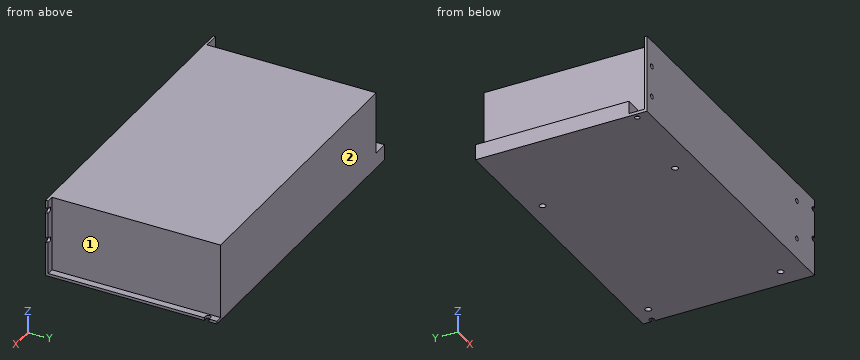
from build123d import *

# Parameters (mm, degrees)
SKETCH_1_W          = 200
SKETCH_1_H          = 110
EXTRUDE_1_DEPTH     = 50
SKETCH_2_R          = 2
CUT_EXTRUDE_1_DEPTH = 10
SKETCH_3_W          = 10
SKETCH_3_H          = 108.5
CUT_EXTRUDE_2_DEPTH = 40
SKETCH_6_W          = 4.5
SKETCH_6_H          = 48.2
CUT_EXTRUDE_5_DEPTH = 108.2
SKETCH_4_R          = 1.5
CUT_EXTRUDE_3_DEPTH = 10
SKETCH_5_R          = 1.6
CUT_EXTRUDE_4_DEPTH = 10
SKETCH_7_W          = 10
SKETCH_7_H          = 10
CUT_EXTRUDE_6_DEPTH = 8.2
SKETCH_8_R          = 1.6
CUT_EXTRUDE_7_DEPTH = 1.8


with BuildPart() as part:
    # 草图1 → 拉伸1 (new body)
    with BuildSketch(Plane.XY):
        with Locations((-22.033224223, 5.842062193)):
            Rectangle(SKETCH_1_W, SKETCH_1_H)
    extrude(amount=EXTRUDE_1_DEPTH)

    # 草图2 → 切除-拉伸1 (cut)
    with BuildSketch(Plane.XY):
        with Locations((-60.533224223, 50.842062193)):
            Circle(SKETCH_2_R)
        with Locations((65.466775777, 50.842062193)):
            Circle(SKETCH_2_R)
        with Locations((-60.533224223, -34.157937807)):
            Circle(SKETCH_2_R)
        with Locations((65.466775777, -34.157937807)):
            Circle(SKETCH_2_R)
    extrude(amount=CUT_EXTRUDE_1_DEPTH, mode=Mode.SUBTRACT)

    # 草图3 → 切除-拉伸2 (cut)
    with BuildSketch(Plane.XY.offset(50)):
        with Locations((-117.033224223, 6.592062193)):
            Rectangle(SKETCH_3_W, SKETCH_3_H)
    extrude(amount=-CUT_EXTRUDE_2_DEPTH, mode=Mode.SUBTRACT)

    # 草图6 → 切除-拉伸5 (cut)
    with BuildSketch(Plane(origin=(0, 60.842062193, 0), x_dir=(-1, 0, 0), z_dir=(0, 1, 0))):
        with Locations((-75.716775777, 25.9)):
            Rectangle(SKETCH_6_W, SKETCH_6_H)
    extrude(amount=-CUT_EXTRUDE_5_DEPTH, mode=Mode.SUBTRACT)

    # 草图4 → 切除-拉伸3 (cut)
    with BuildSketch(Plane.XZ.offset(49.157937807)):
        with Locations(Location((-116.033224223, 13, 0), (0, 0, 270))):
            Circle(SKETCH_4_R)
        with Locations(Location((56.966775777, 13, 0), (0, 0, 270))):
            Circle(SKETCH_4_R)
        with Locations(Location((56.966775777, 38, 0), (0, 0, 270))):
            Circle(SKETCH_4_R)
    extrude(amount=-CUT_EXTRUDE_3_DEPTH, mode=Mode.SUBTRACT)

    # 草图5 → 切除-拉伸4 (cut)
    with BuildSketch(Plane.XZ.offset(49.157937807)):
        with Locations(Location((-116.033224223, 33, 0), (0, 0, 270))):
            Circle(SKETCH_5_R)
        with BuildLine():
            Line((77.966775777, 45), (77.966775777, 41.8))
            Line((77.966775777, 41.8), (76.666775777, 41.8))
            ThreePointArc((76.666775777, 41.8), (75.066775777, 43.4), (76.666775777, 45))
            Line((76.666775777, 45), (77.966775777, 45))
        make_face()
        with BuildLine():
            Line((77.966775777, 22.1), (76.666775777, 22.1))
            ThreePointArc((76.666775777, 22.1), (75.066775777, 23.7), (76.666775777, 25.3))
            Line((76.666775777, 25.3), (77.966775777, 25.3))
            Line((77.966775777, 25.3), (77.966775777, 22.1))
        make_face()
    extrude(amount=-CUT_EXTRUDE_4_DEPTH, mode=Mode.SUBTRACT)

    # 草图7 → 切除-拉伸6 (cut)
    with BuildSketch(Plane.XY.offset(10)):
        with Locations((-117.033224223, -42.657937807)):
            Rectangle(SKETCH_7_W, SKETCH_7_H)
    extrude(amount=-CUT_EXTRUDE_6_DEPTH, mode=Mode.SUBTRACT)

    # 草图8 → 切除-拉伸7 (cut)
    with BuildSketch(Plane(origin=(0, 0, 0), x_dir=(-1, 0, 0), z_dir=(0, 0, -1))):
        with Locations((118.533224223, -41.157937807)):
            Circle(SKETCH_8_R)
        with BuildLine():
            Line((-77.966775777, 55.942062193), (-76.166775777, 55.942062193))
            ThreePointArc((-76.166775777, 55.942062193), (-74.566775777, 54.342062193), (-76.166775777, 52.742062193))
            Line((-76.166775777, 52.742062193), (-77.966775777, 52.742062193))
            Line((-77.966775777, 52.742062193), (-77.966775777, 55.942062193))
        make_face()
    extrude(amount=-CUT_EXTRUDE_7_DEPTH, mode=Mode.SUBTRACT)


solid = part.part
The model under review builds one solid part; all positions refer to its coordinate system, in mm. Face numbers are marked on the shaded views. A direction names the side the tool comes from. Coordinates: 2 decimals unless noted, no trailing zeros. Write each loop counter-clockwise with the first axis right and the second up, starting at its lowest first coordinate (ties: lowest second). Pieces come first, ordered by that corner, then holes. Notation, with made-up numbers: (68.5, -7) - (109.5, -7) arc R18 ccw to (109.5, -1) - close; hole circle Ø7 at (27.5, 19.5). An arc over 180 degrees is marked (long way). Answer as a JSON object with one key per item and string values. Group by question number.
1. Machinability: for the marked faces 1 and 2, which of the approach directions +Z, -Z, +X, -X, +Y, -Y give a long, thin tool a straight path to every point of the face, cutting with its end or side? Answer none if there is none.
2. Add section B-B (z = 7). Give the boundary of the cut face in (x, y).
3. Clearance check with flat-ended pins moving along their axes: pin 1 Ø3 at (x, y) = (-118.53, -41.16) entering from -Z; pin 2 Ø3.5 at (x, y) = (65.47, -34.16) entering from -Z; pin 3 Ø3.5 at (x, y) = (75.5, 27) entering from +Z; pin 4 Ø4 at (y, z) = (-32, 24.5) entering from +X. State where each tip first meets the part, or that it passes through.
4. Add section A-A (z = 19). Give the boundary of the cut face in (x, y).
5. Add section C-C (y = 13). Give the boundary of the cut face in (x, z), plus the area to 3 significant figures.
6. To check wall thickness, follow probe 1 along X at (y, z) = (-41.25, 38); probe 2 along X at (y, z) = (38, 21); probe 3 along Z at (x, y) = (-114, 2). State the ranges of each line that lie inside material, in increasing order.
Findings:
{
 "1": {"face 1": "+Z, +X, +Y", "face 2": "+Z, -Z, +X, -X, +Y"},
 "2": {"outline": "(-122.03, -49.16) - (77.97, -49.16) - (77.97, -47.36) - (73.47, -47.36) - (73.47, 60.84) - (-122.03, 60.84) - (-122.03, -37.66) - (-112.03, -37.66) - (-112.03, -47.66) - (-122.03, -47.66) - close; hole circle Ø4 at (-60.53, -34.16); hole circle Ø4 at (-60.53, 50.84); hole circle Ø4 at (65.47, -34.16); hole circle Ø4 at (65.47, 50.84)"},
 "3": {"pin 1": "through", "pin 2": "z = 10", "pin 3": "z = 1.8", "pin 4": "x = 73.47"},
 "4": {"outline": "(-122.03, -49.16) - (77.97, -49.16) - (77.97, -47.36) - (73.47, -47.36) - (73.47, 60.84) - (-112.03, 60.84) - (-112.03, -47.66) - (-122.03, -47.66) - close"},
 "5": {"outline": "(-122.03, 0) - (77.97, 0) - (77.97, 1.8) - (73.47, 1.8) - (73.47, 50) - (-112.03, 50) - (-112.03, 10) - (-122.03, 10) - close", "area": "9,380 mm²"},
 "6": {"probe 1": "-112.03 to 55.47, 58.47 to 73.47", "probe 2": "-112.03 to 73.47", "probe 3": "0 to 10"}
}
